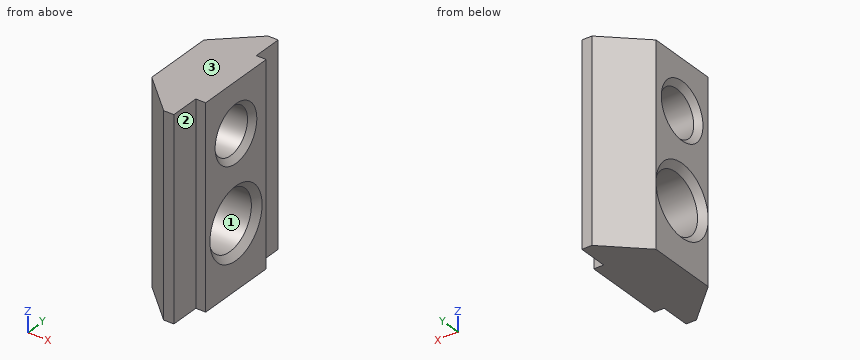
Autodesk Inventor part; units mm, degrees
ref_plane "bolt_XY" through (-4.1, 0, -9.5) normal (1, 0, 0) x (0, 0, -1)
ref_plane "bolt_YZ" through (-4.1, 0, -9.5) normal (0, 0, -1) x (0, 1, 0)
ref_plane "bolt_ZX" through (-4.1, 0, -9.5) normal (0, 1, 0) x (1, 0, 0)
sketch "Sketch_1" plane through (0, 0, 0) normal (0, 0, 1) x (1, 0, 0)
  line L0 (-4.1, -2.5) -> (-1.4191, -5)
  line L1 (-1.4191, -5) -> (-0.7, -5)
  line L2 (-0.7, -5) -> (-0.7, -2.9)
  line L3 (-0.7, -2.9) -> (0, -2.9)
  line L4 (0, -2.9) -> (0, 2.9)
  line L5 (0, 2.9) -> (-0.7, 2.9)
  line L6 (-0.7, 2.9) -> (-0.7, 5)
  line L7 (-0.7, 5) -> (-1.4191, 5)
  line L8 (-1.4191, 5) -> (-4.1, 2.5)
  line L9 (-4.1, 2.5) -> (-4.1, -2.5)
extrude "Extrusion1" add sketch "Sketch_1" against normal blind 14
sketch "Sketch_2" plane through (0, 0, -3.5) normal (0, 0, 1) x (1, 0, 0)
  line L0 (0, 0) -> (-4.1, 0)
  line L1 (-4.1, 0) -> (-4.1, 2)
  line L2 (-4.1, 2) -> (-3.721, 1.621)
  line L3 (-3.721, 1.621) -> (-0.379, 1.621)
  line L4 (-0.379, 1.621) -> (0, 2)
  line L5 (0, 2) -> (0, 0)
  line L6 (0, 0) -> (-4.1, 0)
revolve "Revolution1" cut sketch "Sketch_2" angle 360 about axis through (0, 0, -3.5) along (1, 0, 0)
thread "Thread1"
sketch "Sketch_3" plane through (0, 0, -9.5) normal (0, 0, 1) x (1, 0, 0)
  line L0 (0, 0) -> (-4.1, 0)
  line L1 (-4.1, 0) -> (-4.1, 2.5)
  line L2 (-4.1, 2.5) -> (-3.667, 2.067)
  line L3 (-3.667, 2.067) -> (-0.433, 2.067)
  line L4 (-0.433, 2.067) -> (0, 2.5)
  line L5 (0, 2.5) -> (0, 0)
  line L6 (0, 0) -> (-4.1, 0)
revolve "Revolution2" cut sketch "Sketch_3" angle 360 about axis through (0, 0, -9.5) along (1, 0, 0)
thread "Thread2"
ref_plane "bolt_XY" through (-4.1, 0, -9.5) normal (1, 0, 0) x (0, 0, -1)
ref_plane "bolt_YZ" through (-4.1, 0, -9.5) normal (0, 0, -1) x (0, 1, 0)
ref_plane "bolt_ZX" through (-4.1, 0, -9.5) normal (0, 1, 0) x (1, 0, 0)
ref_plane "frame_XY" through (-0.7, 0, -9.5) normal (1, 0, 0) x (0, 0, -1)
ref_plane "frame_YZ" through (-0.7, 0, -9.5) normal (0, 0, -1) x (0, 1, 0)
ref_plane "frame_ZX" through (-0.7, 0, -9.5) normal (0, 1, 0) x (1, 0, 0)
ref_plane "nut_XY" through (0, 0, -9.5) normal (1, 0, 0) x (0, 0, -1)
ref_plane "nut_YZ" through (0, 0, -9.5) normal (0, 0, -1) x (0, 1, 0)
ref_plane "nut_ZX" through (0, 0, -9.5) normal (0, 1, 0) x (1, 0, 0)
ref_plane "set_screw_XY" through (-4.1, 0, -3.5) normal (1, 0, 0) x (0, 0, -1)
ref_plane "set_screw_YZ" through (-4.1, 0, -3.5) normal (0, 0, -1) x (0, 1, 0)
ref_plane "set_screw_ZX" through (-4.1, 0, -3.5) normal (0, 1, 0) x (1, 0, 0)
properties part number "HNTC5_n" material "鋼、炭素鋼"
Source: CAD feature listing. Evaluate the final solid. Frame: model axes, mm. Face numbers are marked on the shaded views. Give positions to 0.01 mm unless a question says otherwise; leave off trailing zeros. Order: outer loops, then holes, each group sorted by start corner. A loop starts at its lowest first (then second) coordinate and runs counter-clockwise, first axis right, second up. Notation, with made-up numbers: (20, 67.5) -> (29, 67.5) arc R17 cw to (29, 82.5) -> close; hole circle Ø8 at (-36.5, 5.5). An arc over 180 degrees is marked (long way). Use a Markdown table: item, result.
Q1. Section D-D (x = -2.9). Return the cut outline in (y, z), and give its area (3 significant figures).
A:
| item | result |
|---|---|
| outline | (-3.62, -14) -> (3.62, -14) -> (3.62, 0) -> (-3.62, 0) -> close; hole circle Ø4.13 at (0, -9.5); hole circle Ø3.24 at (0, -3.5) |
| area | 79.7 mm^2 |
Q2. Section C-C (z = -12.5). Return the cut outline in (x, y), and give its area (3 significant figures).
A:
| item | result |
|---|---|
| outline | (-4.1, -2.5) -> (-1.42, -5) -> (-0.7, -5) -> (-0.7, -2.9) -> (0, -2.9) -> (0, 2.9) -> (-0.7, 2.9) -> (-0.7, 5) -> (-1.42, 5) -> (-4.1, 2.5) -> close |
| area | 31.4 mm^2 |
Q3. Section B-B (y = 0). Return the cut outline in (x, z), and give its area (3 significant figures).
A:
| item | result |
|---|---|
| outline | (-4.1, -14) -> (0, -14) -> (0, -12) -> (-0.43, -11.57) -> (-3.67, -11.57) -> (-4.1, -12) -> close; (-4.1, -7) -> (-3.67, -7.43) -> (-0.43, -7.43) -> (0, -7) -> (0, -5.5) -> (-0.38, -5.12) -> (-3.72, -5.12) -> (-4.1, -5.5) -> close; (-4.1, -1.5) -> (-3.72, -1.88) -> (-0.38, -1.88) -> (0, -1.5) -> (0, 0) -> (-4.1, 0) -> close |
| area | 26.5 mm^2 |
Q4. First-contact query: P1, Ø0.6, axis at y = -4, z = -8, coming from the +X side; P2, Ø2, axis at x = -3.5, z = -8.5, coming from the +Y side. Flat tips, straight axial feed; report the tip coordinate or a pass-through.
A:
| item | result |
|---|---|
| P1 | x = -0.7 |
| P2 | y = 3.99 |
Q5. Section A-A (z = -3.5). Return the cut outline in (x, y), and give its area (3 significant figures).
A:
| item | result |
|---|---|
| outline | (-4.1, -2.5) -> (-1.42, -5) -> (-0.7, -5) -> (-0.7, -2.9) -> (0, -2.9) -> (0, -2) -> (-0.38, -1.62) -> (-3.72, -1.62) -> (-4.1, -2) -> close; (-4.1, 2) -> (-3.72, 1.62) -> (-0.38, 1.62) -> (0, 2) -> (0, 2.9) -> (-0.7, 2.9) -> (-0.7, 5) -> (-1.42, 5) -> (-4.1, 2.5) -> close |
| area | 17.8 mm^2 |
Q6. Pull-direction query (Z, two-part tool) for the marked faces 1, 2 and 3; classes: +Z half, -Z half, draft (parallel to the pull), parting line (faces both ways), or undercut.
A:
| item | result |
|---|---|
| face 1 | undercut |
| face 2 | draft |
| face 3 | +Z half |
Q7. Material intervals for line 1 (Z direction, x = -2.45, y = 0); line 2 (Z direction, x = -2.85, y = -0.5); line 3 (Y direction, x = -2.65, z = -3.25), sorted ascending. Write a range as [from, to].
A:
| item | result |
|---|---|
| line 1 | [-14, -11.57], [-7.43, -5.12], [-1.88, 0] |
| line 2 | [-14, -11.51], [-7.49, -5.04], [-1.96, 0] |
| line 3 | [-3.85, -1.6], [1.6, 3.85] |
